from build123d import *
from build123d.topology import SkipClean

# Parameters (mm, degrees)
SKETCH1_W                = 41.656
SKETCH1_H                = 45.847
BOSS_EXTRUDE1_DEPTH      = 25.4
SKETCH2_R                = 16.129
CUT_EXTRUDE1_DEPTH       = 25.4
SKETCH3_W                = 2.794
SKETCH3_H                = 7.62
CUT_EXTRUDE2_DEPTH       = 3.81
CUT_EXTRUDE6_START       = -25.4
CUT_EXTRUDE6_DEPTH       = 25.4
CUT_EXTRUDE7_REACH       = 58.4
CUT_EXTRUDE7_END_RADIUS  = 16.129
SKETCH7_R                = 3.048
SKETCH14_W               = 7.43654476
SKETCH14_H               = 2.672753785
SKETCH14_W_2             = 2.524584731
SKETCH14_H_2             = 43.307
CUT_EXTRUDE10_DEPTH      = 2.54
SKETCH17_W               = 45.847
SKETCH17_H               = 22.86
BOSS_EXTRUDE3_DEPTH      = 3.175
CUT_EXTRUDE12_REACH      = 43.576
SKETCH12_R               = 3.048
SKETCH18_W               = 44.831
SKETCH18_H               = 22.86
BOSS_EXTRUDE4_DEPTH      = 1.5875
CUT_EXTRUDE13_DEPTH      = 44.190833792
CUT_EXTRUDE13_DEPTH_BACK = 44.190833792
SKETCH11_R               = 3.048
BOSS_EXTRUDE8_START      = -13.462
BOSS_EXTRUDE8_DEPTH      = 1.462
SKETCH4_R                = 1.778
CUT_EXTRUDE14_DEPTH      = 43.685983001


with BuildPart() as part:
    # Sketch1 → Boss-Extrude1 (new body)
    with BuildSketch(Plane(origin=(0, 0, 0), x_dir=(1, 0, 0), z_dir=(0, 1, 0))):
        Rectangle(SKETCH1_W, SKETCH1_H)
    extrude(amount=BOSS_EXTRUDE1_DEPTH)

    # Sketch2 → Cut-Extrude1 (cut)
    with BuildSketch(Plane(origin=(0, 25.4, 0), x_dir=(1, 0, 0), z_dir=(0, 1, 0))):
        with Locations(Location((0, 2.0955, 0), (0, 0, 270))):
            Circle(SKETCH2_R)
    extrude(amount=-CUT_EXTRUDE1_DEPTH, mode=Mode.SUBTRACT)

    # Sketch3 → Cut-Extrude2 (cut)
    with BuildSketch(Plane(origin=(0, 25.4, 0), x_dir=(1, 0, 0), z_dir=(0, 1, 0))):
        with Locations((18.415, 2.0955)):
            Rectangle(SKETCH3_W, SKETCH3_H)
        with Locations((-18.415, 2.0955)):
            Rectangle(SKETCH3_W, SKETCH3_H)
    extrude(amount=-CUT_EXTRUDE2_DEPTH, mode=Mode.SUBTRACT)

    # Sketch6 → Cut-Extrude6 (cut)
    with BuildSketch(Plane(origin=(0, 25.4, 0), x_dir=(1, 0, 0), z_dir=(0, 1, 0)).offset(CUT_EXTRUDE6_START)):
        with BuildLine():
            ThreePointArc((-2.800771458, 17.979464248), (-1.405734975, 18.163124286), (0, 18.2245))
            ThreePointArc((0, 18.2245), (1.405734975, 18.163124286), (2.800771458, 17.979464248))
            Line((2.800771458, 17.979464248), (2.955144688, 18.854958341))
            ThreePointArc((2.955144688, 18.854958341), (0, 19.1135), (-2.955144688, 18.854958341))
            Line((-2.955144688, 18.854958341), (-2.800771458, 17.979464248))
        make_face()
        with BuildLine():
            Line((0, 18.2245), (0, 2.0955))
            Line((0, 2.0955), (2.800771458, 17.979464248))
            ThreePointArc((2.800771458, 17.979464248), (1.405734975, 18.163124286), (0, 18.2245))
        make_face()
        with BuildLine():
            Line((-2.800771458, 17.979464248), (0, 2.0955))
            Line((0, 2.0955), (0, 18.2245))
            ThreePointArc((0, 18.2245), (-1.405734975, 18.163124286), (-2.800771458, 17.979464248))
        make_face()
    extrude(amount=CUT_EXTRUDE6_DEPTH, mode=Mode.SUBTRACT)

    # Cut-Extrude7: up to this cylinder (the profile starts outside it)
    cut_extrude7_end = Plane(origin=(0, 16.002, -2.0955), z_dir=(0, 1, 0)) * Cylinder(CUT_EXTRUDE7_END_RADIUS, 150.058, mode=Mode.PRIVATE)
    # Sketch7 → Cut-Extrude7 (cut, up to the surface)
    with BuildSketch(Plane.XY.offset(22.9235), mode=Mode.PRIVATE) as cut_extrude7_sk1:
        with Locations((0, 16.002)):
            Circle(SKETCH7_R)
    cut_extrude7_tool1 = extrude(cut_extrude7_sk1.sketch, amount=-CUT_EXTRUDE7_REACH, mode=Mode.PRIVATE) - cut_extrude7_end
    add(cut_extrude7_tool1.solids().sort_by_distance((0, 16.002, 22.9235))[0], mode=Mode.SUBTRACT)

    # Sketch14 → Cut-Extrude10 (cut)
    with BuildSketch(Plane(origin=(0, 25.4, 0), x_dir=(1, 0, 0), z_dir=(0, 1, 0))):
        with Locations((0, -20.25731759)):
            Rectangle(SKETCH14_W, SKETCH14_H)
        Polygon((20.828, -22.9235), (20.828, 20.3835), (18.288, 20.3835), (18.288, 5.9055), (19.812, 5.9055), (19.812, -1.7145), (18.288, -1.7145), (18.288, -22.9235), align=None)
        Polygon((20.828, 22.9235), (-20.828, 22.9235), (-20.828, 20.3835), (-18.303415269, 20.3835), (18.288, 20.3835), (20.828, 20.3835), align=None)
        with Locations((-19.565707635, -1.27)):
            Rectangle(SKETCH14_W_2, SKETCH14_H_2)
    extrude(amount=-CUT_EXTRUDE10_DEPTH, mode=Mode.SUBTRACT)

    # Sketch17 → Boss-Extrude3 (add)
    with BuildSketch(Plane(origin=(20.828, 0, 0), x_dir=(0, 0, -1), z_dir=(1, 0, 0))):
        with Locations((0, 11.43)):
            Rectangle(SKETCH17_W, SKETCH17_H)
    extrude(amount=BOSS_EXTRUDE3_DEPTH)

    # Cut-Extrude12: up to this plane
    cut_extrude12_end = Plane(origin=(24.003, 0, 0), z_dir=(1, 0, 0))
    # Sketch12 → Cut-Extrude12 (cut, up to the surface)
    with BuildSketch(Plane(origin=(0.914260378, 0, -0.535980498), x_dir=(-0.50574390925612, 0, -0.862683660590797), z_dir=(0.862683660590797, 0, -0.50574390925612)), mode=Mode.PRIVATE) as cut_extrude12_sk1:
        with Locations(Location((1.807753611, 16.002, 0), (0, 0, 180))):
            Circle(SKETCH12_R)
    cut_extrude12_tool1 = split(extrude(cut_extrude12_sk1.sketch, amount=CUT_EXTRUDE12_REACH, mode=Mode.PRIVATE), bisect_by=cut_extrude12_end, keep=Keep.BOTH, mode=Mode.PRIVATE)
    add(cut_extrude12_tool1.solids().sort_by_distance((0, 16.002, -2.0955))[0], mode=Mode.SUBTRACT)

    # Sketch18 → Boss-Extrude4 (add)
    with BuildSketch(Plane(origin=(0, 0, -22.9235), x_dir=(-1, 0, 0), z_dir=(0, 0, -1))):
        with Locations((-1.5875, 11.43)):
            Rectangle(SKETCH18_W, SKETCH18_H)
    extrude(amount=BOSS_EXTRUDE4_DEPTH)

    # Sketch11 → Cut-Extrude13 (cut, two sides: drawn at the far end of the back side and taken through both)
    with BuildSketch(Plane(origin=(-0.914260378, 0, -1.559519502), x_dir=(0.862683660590797, 0, -0.50574390925612), z_dir=(0.50574390925612, 0, 0.862683660590797)).offset(-CUT_EXTRUDE13_DEPTH_BACK)):
        with Locations((1.059786362, 16.002)):
            Circle(SKETCH11_R)
    extrude(amount=CUT_EXTRUDE13_DEPTH + CUT_EXTRUDE13_DEPTH_BACK, mode=Mode.SUBTRACT)

    # Boss-Extrude8: read off the stored shape, not the designer's step
    # Boss-Extrude8 outline → Boss-Extrude8 (add)
    with SkipClean():  # the faces are left unmerged after this step: merging them gives an invalid solid
        with BuildSketch(Plane.XZ.offset(BOSS_EXTRUDE8_START)):
            with BuildLine():
                ThreePointArc((13.119762317, 16.952399563), (11.697350877, 17.857510386), (10.212785134, 18.656600154))
                Line((10.212785134, 18.656600154), (6.659027379, 12.594700658))
                ThreePointArc((6.659027379, 12.594700658), (8.157143512, 11.818724762), (9.566004562, 10.890500066))
                Line((9.566004562, 10.890500066), (13.119762317, 16.952399563))
            make_face()
            with BuildLine():
                ThreePointArc((-6.659027379, -16.785700658), (-8.157143512, -16.009724762), (-9.566004562, -15.081500066))
                Line((-9.566004562, -15.081500066), (-13.119762317, -21.143399563))
                ThreePointArc((-13.119762317, -21.143399563), (-11.697350877, -22.048510386), (-10.212785134, -22.847600154))
                Line((-10.212785134, -22.847600154), (-6.659027379, -16.785700658))
            make_face()
            with BuildLine():
                Line((20.752100154, -12.308285134), (14.690200658, -8.754527379))
                ThreePointArc((14.690200658, -8.754527379), (13.914224762, -10.252643512), (12.986000066, -11.661504562))
                Line((12.986000066, -11.661504562), (19.047899563, -15.215262317))
                ThreePointArc((19.047899563, -15.215262317), (19.953010386, -13.792850877), (20.752100154, -12.308285134))
            make_face()
            with BuildLine():
                ThreePointArc((1.684845394, 20.972051604), (0, 21.0335), (-1.684845394, 20.972051604))
                Line((-1.684845394, 20.972051604), (-1.684845394, 13.945258617))
                ThreePointArc((-1.684845394, 13.945258617), (0, 14.0335), (1.684845394, 13.945258617))
                Line((1.684845394, 13.945258617), (1.684845394, 20.972051604))
            make_face()
        extrude(amount=BOSS_EXTRUDE8_DEPTH)

    # Sketch4 → Cut-Extrude14 (cut, through all)
    with SkipClean():  # the faces are left unmerged after this step: merging them gives an invalid solid
        with BuildSketch(Plane(origin=(0, 25.4, 0), x_dir=(1, 0, 0), z_dir=(0, 1, 0))):
            with Locations(Location((-16.002, -13.9065, 0), (0, 0, 270))):
                Circle(SKETCH4_R)
            with Locations(Location((-16.002, 18.0975, 0), (0, 0, 90))):
                Circle(SKETCH4_R)
            with Locations(Location((16.002, 18.0975, 0), (0, 0, 270))):
                Circle(SKETCH4_R)
            with Locations(Location((16.002, -13.9065, 0), (0, 0, 90))):
                Circle(SKETCH4_R)
        extrude(amount=-CUT_EXTRUDE14_DEPTH, mode=Mode.SUBTRACT)


solid = part.part
Source: CAD feature listing. Evaluate the final solid. Frame: model axes, mm. A direction names the side the tool comes from. Round coordinates to 2 decimals unless told otherwise and drop trailing zeros. Loops run counter-clockwise (first coordinate to the right, second up) from the corner with the lowest first, then second, coordinate; pieces in that order, holes last. Notation, with made-up numbers: M 86,41.25 L 96,41.25 A28 cw 96,71.25 Z; hole C 10.5,47.25 d4. An arc over 180 degrees is marked long. Answer as CSV lines item,"result".
Q1. Cut plane A-A (y = 17). Return the cut outline in (x, z).
Verdict:
outline,"M -20.83,-24.51 L -16.48,-24.51 L -10.51,-14.33 A16.13 cw -2.88,13.77 L -2.88,22.92 L -20.83,22.92 Z; M -9.8,-24.51 L 24,-24.51 L 24,-19.51 L 12.23,-12.61 A16.13 cw 2.8,-17.98 L 2.96,-18.85 A17.02 cw -2.96,-18.85 L -2.8,-17.98 A16.13 cw -5.54,-17.24 Z; M 2.88,13.77 A16.13 cw 5.54,13.05 L 11.33,22.92 L 2.88,22.92 Z; M 10.51,10.14 A16.13 cw 15.15,-7.64 L 24,-12.83 L 24,22.92 L 18.01,22.92 Z; hole C -16,-18.1 d3.56; hole C -16,13.91 d3.56; hole C 16,-18.1 d3.56; hole C 16,13.91 d3.56"
Q2. Pull-direction query (X, two-part tool) for faces 1 (the face through (20, 22.86, -6)), 2 (the face through (0.042, 12.522, -19.113)), 3 (the face through (18.288, 24, -13)); classes: +X half, -X half, draft (parallel to the pull), parting line (faces both ways), or undercut.
Verdict:
face 1,"draft"
face 2,"undercut"
face 3,"+X half"
Q3. Reachability of faces 4 (the face through (17, 13.462, -12)), 5 (the face through (0, 24, -20.384)), 6 (the face through (18.288, 24, 12)), 7 (the face through (-18.303, 24, 12)), 8 (the face through (18, 21.59, -2)) from +Z, -Z, +X, -X, +Y, -Y: full face, straight path, thin tool, end or side. Return the list, or none.
Verdict:
face 4,"none"
face 5,"-Z, +X, -X, +Y"
face 6,"+Z, -Z, +X, +Y"
face 7,"+Z, -Z, -X, +Y"
face 8,"+Y"
Q4. Cut plane B-B (x = -4.5). Return the cut outline in (y, z).
Verdict:
outline,"M 0,-24.51 L 22.86,-24.51 L 22.86,-20.38 L 25.4,-20.38 L 25.4,-17.58 L 0,-17.58 Z; M 0,13.39 L 25.4,13.39 L 25.4,22.92 L 0,22.92 Z"
Q5. Cut plane D-D (z = 1). Return the cut outline in (x, y), plus the area to 3 significant figures.
Verdict:
outline,"M -20.83,0 L -15.83,0 L -15.83,25.4 L -17.02,25.4 L -17.02,21.59 L -19.81,21.59 L -19.81,22.86 L -20.83,22.86 Z; M 15.83,0 L 24,0 L 24,22.86 L 19.81,22.86 L 19.81,21.59 L 17.02,21.59 L 17.02,25.4 L 15.83,25.4 Z"
area,"300 mm^2"
Q6. Line query: line 1 along X through (y, z) = (22.5, -2); line 2 along Z through (x, y) = (16.5, 20.25); line 3 along Z through (x, y) = (-0.5, 11.5). Output: solid intervals per line, ascending.
Verdict:
line 1,"x = -20.83 to -19.81, -17.02 to -16.13, 16.13 to 17.02, 19.81 to 24"
line 2,"z = -24.51 to -19.8, -16.39 to 12.2, 15.61 to 22.92"
line 3,"z = -24.51 to -19.11, 14.03 to 22.92"
Q7. Cut plane C-C (x = 0). Return the cut outline in (y, z).
Verdict:
outline,"M 0,-24.51 L 22.86,-24.51 L 22.86,-20.38 L 25.4,-20.38 L 25.4,-19.11 L 0,-19.11 Z; M 0,14.03 L 13.46,14.03 L 13.46,21.03 L 12.95,21.03 L 12.95,22.92 L 0,22.92 Z; M 19.05,14.03 L 25.4,14.03 L 25.4,18.92 L 22.86,18.92 L 22.86,21.59 L 25.4,21.59 L 25.4,22.92 L 19.05,22.92 Z"
Q8. Contact query for flat-ended pins moving along their axis: pin 1 (8 mm diameter, centred on x = -5, z = -10.5, fed in from -Y); pin 2 (0.8 mm diameter, centred on x = 19, z = -3, fed in from +Y); pin 3 (1.3 mm diameter, centred on y = 24, z = 20.5, fed in from +X); pin 4 (0.8 mm diameter, centred on x = 18.5, y = 24, fed in from -Z). Output: stop coordinate, or through.
Verdict:
pin 1,"passes through"
pin 2,"stops at y = 21.59"
pin 3,"stops at x = 18.29"
pin 4,"stops at z = -20.38"
